```python
from build123d import *

# Parameters (mm, degrees)
F0_W     = 6
F0_H     = 0.3
F1_DEPTH = 7
F3_DEPTH = 2
F4_R     = 2


# Not quite as in the source:
# - a feature names something its author has since deleted; it is built from what else it names


with BuildPart() as f1:
    # F0 (on Top) → F1 (new body)
    with BuildSketch(Plane.XY):
        Polygon((0, -4), (-3.5, -0.5), (-3.5, -65.5), (-23.5, -65.5), (-23.5, -70.5), (-17.5, -70.5), (-3.6, -70.5), (-3.6, -67.4), (3.6, -67.4), (3.6, -70.5), (17.5, -70.5), (23.5, -70.5), (23.5, -65.5), (3.5, -65.5), (3.5, -0.5), align=None)
        with Locations((-20.5, -70.65)):
            Rectangle(F0_W, F0_H)
        with Locations((20.5, -70.65)):
            Rectangle(F0_W, F0_H)
        Polygon((-20, 16), (-3.5, -0.5), (0, -4), (3.5, -0.5), (20, 16), (0, 36), align=None)
    extrude(amount=F1_DEPTH)

    # F2 (on face) → F3 (cut)
    with BuildSketch(Plane.XY.offset(7)):
        Polygon((0, 33.1715728753), (-17.1715728753, 16), (0, -1.1715728753), (17.1715728753, 16), align=None)
    extrude(amount=-F3_DEPTH, mode=Mode.SUBTRACT)

    # F4
    f4_edges = [f1.edges().sort_by_distance(p)[0] for p in [
        (3.5, -65.5, 3.5),
        (-3.5, -65.5, 3.5),
        (-23.5, -65.5, 3.5),
        (23.5, -65.5, 3.5),
        (-23.5, -70.8, 3.5),
        (23.5, -70.8, 3.5),
        (20, 16, 3.5),
        (0, 36, 3.5),
        (-20, 16, 3.5),
        (3.5, -0.5, 3.5),
        (-3.5, -0.5, 3.5),
    ]]
    fillet(f4_edges, radius=F4_R)


solid = f1.part
```
For this review, take the finished solid that the model builds, in its own axes (mm). A direction names the side the tool comes from. Coordinates: 2 decimals unless noted, no trailing zeros. Write each loop counter-clockwise with the first axis right and the second up, starting at its lowest first coordinate (ties: lowest second). Pieces come first, ordered by that corner, then holes. Notation, with made-up numbers: (13, 39.5) -> (35, 39.5) arc R6 ccw to (35, 50.5) -> close; hole circle Ø3 at (56.5, 81). An arc over 180 degrees is marked (long way). Put each result on its own line as item: value.
Q1. The part is to be moulded in two halves that separate along X. For faces 5 (the cylindrical face through (-22.9, -66.07, 3.55)), 6 (the flat face through (-3.6, -69, 3)), 7 (the flat face through (14, -65.5, 3)), say which applies: +X half, -X half, draft (parallel to the pull), parting line (faces both ways), or undercut.
From the geometry:
face 5: -X half
face 6: undercut
face 7: draft
Q2. Take a section at C-C, the plane y = 29. State the section outline as (x, z) points, then the cut area to 3 significant figures.
From the geometry:
outline: (-7, 0) -> (7, 0) -> (7, 7) -> (4.17, 7) -> (4.17, 5) -> (-4.17, 5) -> (-4.17, 7) -> (-7, 7) -> close
area: 81.3 mm2
Q3. Wall thickness on L1, parallel to Y at x = 7, z = 5.5; L2, parallel to Z at x = -8, y = 21.5; L3, parallel to X at y = -3, z = 2: over which ranges is each line inside the solid? List them lowest first.
From the geometry:
L1: y = -70.5 to -65.5, 3 to 5.83, 26.17 to 29
L2: z = 0 to 5
L3: x = -3.5 to 3.5
Q4. Tool access review of faces 1 (the flat face through (-11, 7, 3)), 2 (the flat face through (0, -67.4, 3)), 3 (the flat face through (3.5, -33, 3)), 4 (the flat face through (8.466, 7.294, 6.014)): name each direction out of +Z, -Z, +X, -X, +Y, -Y from which nothing blocks a thin tool from reaching the whole face with its end or side.
From the geometry:
face 1: +Z, -Z, -X
face 2: +Z, -Z, -Y
face 3: +Z, -Z, +X
face 4: +Z
Q5. Take a section at B-B, the plane x = -16. State the section outline as (y, z) points.
From the geometry:
outline: (-70.5, 0) -> (-65.5, 0) -> (-65.5, 7) -> (-70.5, 7) -> close; (12, 0) -> (20, 0) -> (20, 7) -> (17.17, 7) -> (17.17, 5) -> (14.83, 5) -> (14.83, 7) -> (12, 7) -> close
Q6. Clearance check with flat-ended pins moving along their axes: pin 1 Ø1.5 at (y, z) = (-18.5, 5.5) entering from -X; pin 2 Ø2 at (y, z) = (-44, 3.5) entering from +X; pin 3 Ø3 at (y, z) = (2, 2.5) entering from -X. State where each tip first meets the part, or that it passes through.
From the geometry:
pin 1: stops at x = -3.5
pin 2: stops at x = 3.5
pin 3: stops at x = -7.5
Q7. Take a section at D-D, the plane x = -8.5. State the section outline as (y, z) points, then the cut area to 3 significant figures.
From the geometry:
outline: (-70.5, 0) -> (-65.5, 0) -> (-65.5, 7) -> (-70.5, 7) -> close; (4.5, 0) -> (27.5, 0) -> (27.5, 7) -> (24.67, 7) -> (24.67, 5) -> (7.33, 5) -> (7.33, 7) -> (4.5, 7) -> close
area: 161 mm2
